Source: CAD feature listing. Evaluate the final solid. Frame: model axes, mm. A direction names the side the tool comes from. Round coordinates to 2 decimals unless told otherwise and drop trailing zeros. Write each loop counter-clockwise with the first axis right and the second up, starting at its lowest first coordinate (ties: lowest second). Pieces come first, ordered by that corner, then holes. Notation, with made-up numbers: (40.5, 63) -> (96.5, 63) arc R23 ccw to (96.5, 98) -> close; hole circle Ø10 at (29.5, 87). An arc over 180 degrees is marked (long way). Put each result on its own line as item: value.
```python
from build123d import *

# Parameters (mm, degrees)
F0_W     = 44.45
F0_H     = 20.6375
F0_R     = 7.9375
F1_DEPTH = 1.5875
F2_DEPTH = 14.2875
F3_R     = 0.5


with BuildPart() as f1:
    # F0 (on Top) → F1 (new body)
    with BuildSketch(Plane.XY):
        Rectangle(F0_W, F0_H)
        with Locations((-11.551156, 0)):
            Circle(F0_R, mode=Mode.SUBTRACT)
        with Locations((11.551156, 0)):
            Circle(F0_R, mode=Mode.SUBTRACT)
        with Locations((-11.551156, 0)):
            Circle(F0_R)
        with Locations((11.551156, 0)):
            Circle(F0_R)
    extrude(amount=F1_DEPTH)

    # F0 (on Top) → F2 (join)
    with BuildSketch(Plane.XY):
        with Locations((-11.551156, 0)):
            Circle(F0_R)
        with Locations((11.551156, 0)):
            Circle(F0_R)
    extrude(amount=F2_DEPTH)

    # F3
    f3_edges = [f1.edges().sort_by_distance(p)[0] for p in [
        (-19.488656, 0, 14.2875),
        (3.613656, 0, 14.2875),
    ]]
    fillet(f3_edges, radius=F3_R)


solid = f1.part
```
Q1. Pin query (flat end, axial travel): pin 1 (1.5 mm diameter, centred on y = 4.5, z = 5.5, fed in from +X); pin 2 (8 mm diameter, centred on y = 8, z = 12.5, fed in from +X); pin 3 (3 mm diameter, centred on y = -3.5, z = 5.5, fed in from -X). Return the tip coordinate at first contact, or that it passes through.
Ans:
pin 1: stops at x = 18.55
pin 2: stops at x = 18.41
pin 3: stops at x = -19.23
Q2. Cut plane C-C on y = 8.75. Output: boundary loops of the cut face in (x, z) (1 decimal), and give its area (3 significant figures).
Ans:
outline: (-22.2, 0) -> (22.2, 0) -> (22.2, 1.6) -> (-22.2, 1.6) -> close
area: 70.6 mm^2
Q3. Draft query along X for faces 1 (the flat face through (0, 0, 1.588)), 2 (the flat face through (11, 0, 14.288)), 3 (the flat face through (22.225, 0, 1)). Return one class per face: +X half, -X half, draft (parallel to the pull), parting line (faces both ways), or undercut.
Ans:
face 1: undercut
face 2: draft
face 3: +X half
Q4. Cut plane B-B on z = 6.75. Output: boundary loops of the cut face in (x, y) (1 decimal).
Ans:
outline: circle Ø15.9 at (-11.6, 0); circle Ø15.9 at (11.6, 0)
Q5. Cut plane A-A on y = 0. Output: boundary loops of the cut face in (x, z) (1 decimal), and give its area (3 significant figures).
Ans:
outline: (-22.2, 0) -> (22.2, 0) -> (22.2, 1.6) -> (19.5, 1.6) -> (19.5, 13.8) arc R0.5 ccw to (19, 14.3) -> (4.1, 14.3) arc R0.5 ccw to (3.6, 13.8) -> (3.6, 1.6) -> (-3.6, 1.6) -> (-3.6, 13.8) arc R0.5 ccw to (-4.1, 14.3) -> (-19, 14.3) arc R0.5 ccw to (-19.5, 13.8) -> (-19.5, 1.6) -> (-22.2, 1.6) -> close
area: 474 mm^2
Q6. Material intervals for line 1 (Z direction, x = 6, y = -8.25); line 2 (X direction, y = 1.5, z = 8.25); line 3 (X direction, y = -4.25, z = 11.5) (3 decimals), sorted ascending. Write a range as [from, to].
Ans:
line 1: z = [0, 1.59]
line 2: x = [-19.35, -3.76], [3.76, 19.35]
line 3: x = [-18.255, -4.847], [4.847, 18.255]
Q7. Reachability of faces 4 (the cylindrical face through (3.62, 0.35, 7.6)), 5 (the flat face through (-12, 0, 14.288)) from +Z, -Z, +X, -X, +Y, -Y: full face, straight path, thin tool, end or side. Return the list, or none.
Ans:
face 4: +Z
face 5: +Z, +X, -X, +Y, -Y
